from build123d import *

# Parameters (mm, degrees)
SKETCH1_W           = 109.22
SKETCH1_H           = 40.64
SKETCH1_W_2         = 104.14
SKETCH1_H_2         = 35.56
BOSS_EXTRUDE1_DEPTH = 2.54
SKETCH2_W           = 2.54
SKETCH2_H           = 2.54
BOSS_EXTRUDE2_DEPTH = 2.54
SKETCH4_W           = 2.54
SKETCH4_H           = 2.54
BOSS_EXTRUDE3_DEPTH = 2.54
SKETCH6_W           = 2.54
SKETCH6_H           = 2.54
BOSS_EXTRUDE4_DEPTH = 2.54


with BuildPart() as part:
    # Sketch1 → Boss-Extrude1 (new body)
    with BuildSketch(Plane.XY):
        with Locations((-54.61, 20.32)):
            Rectangle(SKETCH1_W, SKETCH1_H)
        with Locations((-54.61, 20.32)):
            Rectangle(SKETCH1_W_2, SKETCH1_H_2, mode=Mode.SUBTRACT)
    extrude(amount=BOSS_EXTRUDE1_DEPTH)

    # Sketch2 → Boss-Extrude2 (add)
    with BuildSketch(Plane(origin=(0, 0, 0), x_dir=(-1, 0, 0), z_dir=(0, 0, -1))):
        with Locations((90.17, 39.37)):
            Rectangle(SKETCH2_W, SKETCH2_H)
        with Locations((90.17, 1.27)):
            Rectangle(SKETCH2_W, SKETCH2_H)
    boss_extrude2 = extrude(amount=BOSS_EXTRUDE2_DEPTH)

    # Mirror1: Boss-Extrude2 across plane
    add(boss_extrude2.mirror(Plane.XY.offset(1.27)))

    # Sketch4 → Boss-Extrude3 (add)
    with BuildSketch(Plane(origin=(0, 40.64, 0), x_dir=(1, 0, 0), z_dir=(0, 1, 0))):
        with Locations((-90.17, 1.27)):
            Rectangle(SKETCH4_W, SKETCH4_H)
        with Locations((-90.17, -3.81)):
            Rectangle(SKETCH4_W, SKETCH4_H)
    boss_extrude3 = extrude(amount=BOSS_EXTRUDE3_DEPTH)

    # Sketch6 → Boss-Extrude4 (add)
    with BuildSketch(Plane(origin=(0, 38.1, 0), x_dir=(-1, 0, 0), z_dir=(0, -1, 0))):
        with Locations((90.17, 1.27)):
            Rectangle(SKETCH6_W, SKETCH6_H)
        with Locations((90.17, -3.81)):
            Rectangle(SKETCH6_W, SKETCH6_H)
    boss_extrude4 = extrude(amount=BOSS_EXTRUDE4_DEPTH)

    # Mirror3: Boss-Extrude3, Boss-Extrude4 across plane
    add(boss_extrude3.mirror(Plane(origin=(0, 20.32, 0), x_dir=(0, 0, 1), z_dir=(0, -1, 0))))
    add(boss_extrude4.mirror(Plane(origin=(0, 20.32, 0), x_dir=(0, 0, 1), z_dir=(0, -1, 0))))


solid = part.part
Part model, mm, in its own coordinate system. A direction names the side the tool comes from. Coordinates: 2 decimals unless noted, no trailing zeros. Loops run counter-clockwise (first coordinate to the right, second up) from the corner with the lowest first, then second, coordinate; pieces in that order, holes last. Notation, with made-up numbers: (48.5, -8) - (100.5, -8) arc R15 ccw to (100.5, 13) - close; hole circle Ø2 at (73.25, -5.75). An arc over 180 degrees is marked (long way). Write each question's results on one line, items separated by ' | '. Start each with the question number.
Q1. Probe line 1 along Y through (x, z) = (-81.5, 1.75); line 2 along X through (y, z) = (18.5, 0.5); line 3 along X through (y, z) = (40, 4.5). List the from-to ranges inside material, lowest first.
Q2. Slice it at C-C on y = 39.5. Give the cut face in (x, z), and give its area (3 significant figures).
Q3. Which spindle directions (+Z, -Z, +X, -X, +Y, -Y) get a long thin tool onto all of the face, cutting with end or side? Do faces 4 (the flat face through (-90, 35.56, 4)), 5 (the flat face through (-88.9, 39, -1)), 6 (the flat face through (-90, 37, 2.54)), 7 (the flat face through (-90, -1, 0)). Say none if no direction does.
Q4. Slice it at B-B on z = 4. Give the cut face in (x, y).
Q5. Two-plate mould, pull along Y, no slides. Class faces 1 (the flat face through (-55, 2.54, 1)), 2 (the flat face through (-90, 43.18, -1)), 3 (the flat face through (-91.44, 1, -1)): +Y half, -Y half, draft (parallel to the pull), parting line (faces both ways), or undercut.
Q6. Drop flat-ended pins along their axis: pin 1 Ø1.3 at (x, z) = (-37.5, 2) entering from -Y; pin 2 Ø3 at (x, z) = (-21.5, 3.5) entering from +Y; pin 3 Ø2 at (y, z) = (1, 4) entering from +X. Give the stop position or say it passes through.
Q7. Slice it at A-A on y = 17. Give the cut face in (x, z).
Answer:
1) line 1: y = 0 to 2.54, 38.1 to 40.64 | line 2: x = -109.22 to -106.68, -2.54 to 0 | line 3: x = -91.44 to -88.9
2) outline: (-109.22, 0) - (-91.44, 0) - (-91.44, -2.54) - (-88.9, -2.54) - (-88.9, 0) - (0, 0) - (0, 2.54) - (-88.9, 2.54) - (-88.9, 5.08) - (-91.44, 5.08) - (-91.44, 2.54) - (-109.22, 2.54) - close | area: 290 mm2
3) face 4: +Z, -Z, +X, -X | face 5: -Z, +X, +Y, -Y | face 6: none | face 7: +X, -X, -Y
4) outline: (-91.44, -2.54) - (-88.9, -2.54) - (-88.9, 5.08) - (-91.44, 5.08) - close; (-91.44, 35.56) - (-88.9, 35.56) - (-88.9, 43.18) - (-91.44, 43.18) - close
5) face 1: undercut | face 2: +Y half | face 3: draft
6) pin 1: stops at y = 0 | pin 2: stops at y = 40.64 | pin 3: stops at x = -88.9
7) outline: (-109.22, 0) - (-106.68, 0) - (-106.68, 2.54) - (-109.22, 2.54) - close; (-2.54, 0) - (0, 0) - (0, 2.54) - (-2.54, 2.54) - close
